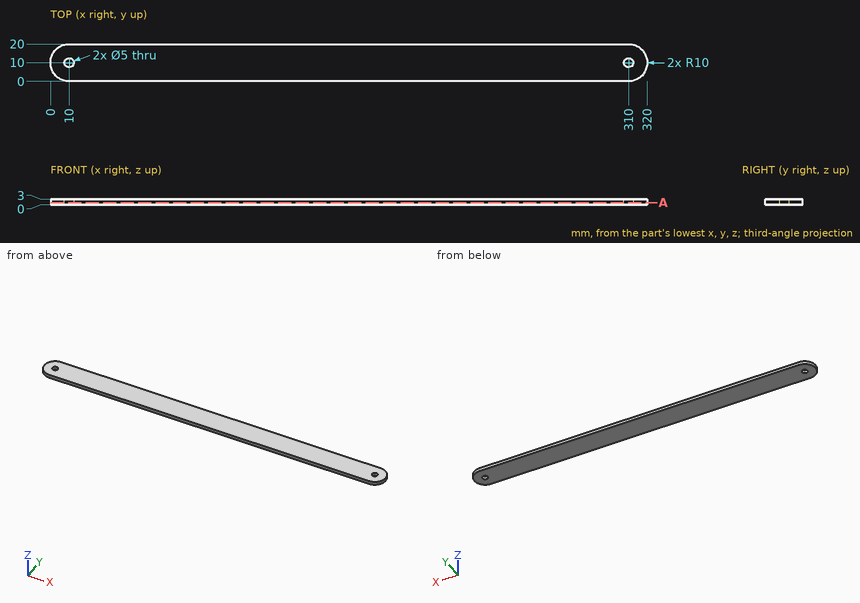
Can you work these out from the drawing? Everything is in mm from the part's minimum corner. Round coordinates to 2 decimals unless told otherwise and drop trailing zeros. Order: outer loops, then holes, each group sorted by start corner. A loop starts at its lowest first (then second) coordinate and runs counter-clockwise, first axis right, second up. Notation, with made-up numbers: (-19.5, -31) -> (-1.5, -31) arc R8 cw to (-1.5, -26) -> close; hole circle Ø3 at (-19, 22). An arc over 180 degrees is marked (long way). Return JSON: item names as keys, results as strings. Group by question number.
1. Will these pins go through, and if not, where does the flat tip stop? pin 1 (1 mm diameter, centred on y = 17, z = 0.5, fed in from -X); pin 2 (6.5 mm diameter, centred on x = 10, y = 10, fed in from +Z); pin 3 (4.5 mm diameter, centred on x = 310, y = 10, fed in from -Z).
2. If we section it at A-A, the plane z = 1.15: Write out the boundary of the cut face in (x, y).
3. I need wall thicknesses on line 1 (Y direction, x = 10, z = 2); line 2 (X direction, y = 1.75, z = 1.65); line 3 (X direction, y = 4.25, z = 0.85). Which ranges of each line are inside material? Lowest first, please. Write a range as [from, to].
Output values:
{
 "1": {"pin 1": "x = 2.4", "pin 2": "z = 3", "pin 3": "through"},
 "2": {"outline": "(10, 0) -> (310, 0) arc R10 ccw to (310, 20) -> (10, 20) arc R10 ccw to start; hole circle Ø5 at (10, 10); hole circle Ø5 at (310, 10)"},
 "3": {"line 1": "[0, 7.5], [12.5, 20]", "line 2": "[4.35, 315.65]", "line 3": "[1.82, 318.18]"}
}
